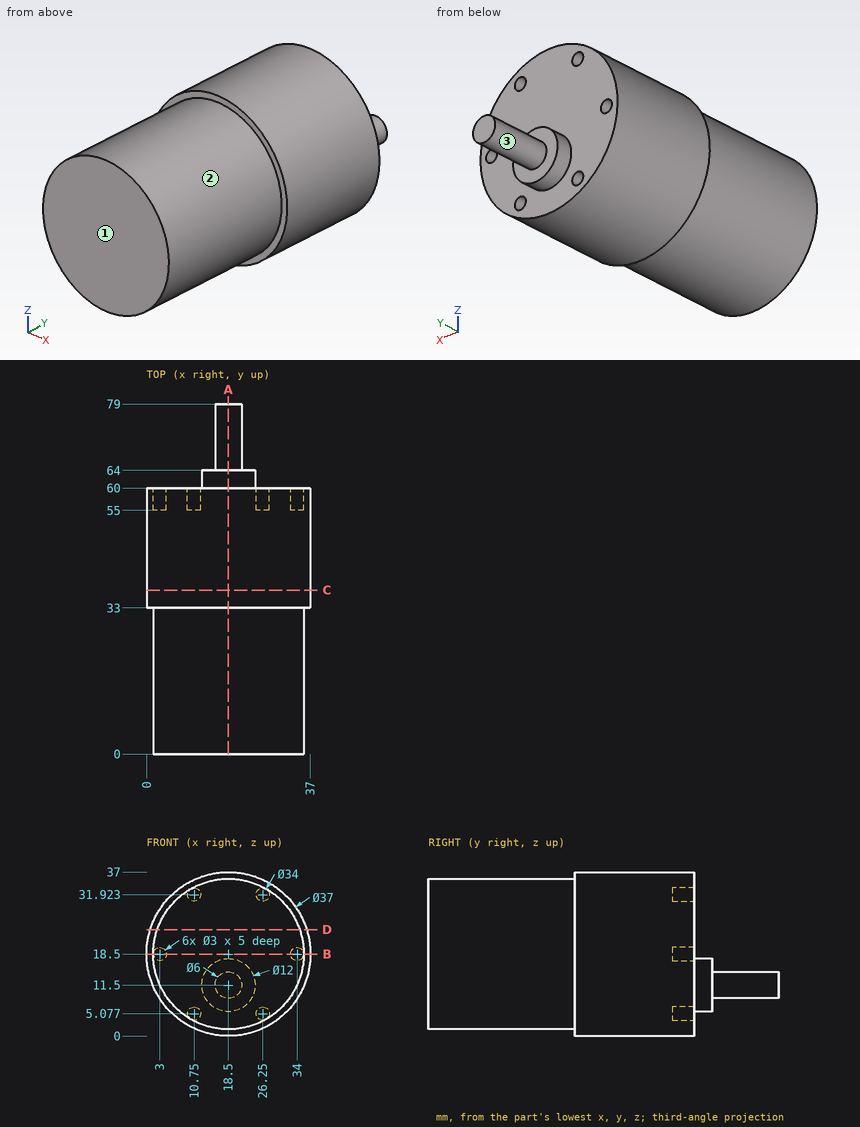
Could you check a few things on this drawing? It's one solid part, dimensions in mm from its lowest x, y, z. A direction names the side the tool comes from. Give positions to 0.01 mm unless a question says otherwise; leave off trailing zeros. Loops run counter-clockwise (first coordinate to the right, second up) from the corner with the lowest first, then second, coordinate; pieces in that order, holes last. Notation, with made-up numbers: M 21,-3.5 L 33,-3.5 A19 ccw 33,1.5 Z; hole C 75.5,49 d2. An arc over 180 degrees is marked long. One line per question, with ' | ' between items. Start each with the question number.
Q1. If we section it at A-A (x = 18.5): Please give me the cut outline in (y, z), plus the area to 3 significant figures.
Q2. If I drill on line 1 (X direction, y = 57.45, z = 18.5); line 2 (Z direction, x = 10, y = 57) (1 decimal); line 3 (Y direction, x = 9.5, z = 25), over which ranges is the centre line in solid material (lowest first)? Write a range as from..to.
Q3. If we section it at D-D (z = 24): Please give me the cut outline in (x, y) (1 decimal), plus the area to 3 significant figures.
Q4. If we section it at B-B (z = 18.5): Please give me the cut outline in (x, y).
Q5. For the marked faces 1, 2 and 3, which set-ups out of +Z, -Z, +X, -X, +Y, -Y let a thin tool reach every point of the face, with its end or its side?
Q6. For pin 1 Ø2.5 at (x, z) = (26, 32.5) entering from +Y; pin 2 Ø1.5 at (x, z) = (3, 19) entering from +Y; pin 3 Ø12 at (y, z) = (37.5, 8.5) entering from -X, each with a flat end and sliding along its axis, tell me the tip position at first contact or that it passes through.
Q7. If we section it at C-C (y = 37): Please give me the cut outline in (x, z), plus the area to 3 significant figures.
Computed:
1) outline: M 0,1.5 L 33,1.5 L 33,0 L 60,0 L 60,5.5 L 64,5.5 L 64,8.5 L 79,8.5 L 79,14.5 L 64,14.5 L 64,17.5 L 60,17.5 L 60,37 L 33,37 L 33,35.5 L 0,35.5 Z | area: 2,260 mm²
2) line 1: x = 0..1.5, 4.5..32.5, 35.5..37 | line 2: z = 2.1..3.8, 6.4..30.6, 33.2..34.9 | line 3: y = 0..60
3) outline: M 0.8,33 L 2.4,33 L 2.4,0 L 34.6,0 L 34.6,33 L 36.2,33 L 36.2,60 L 0.8,60 Z | area: 2,020 mm²
4) outline: M 0,33 L 1.5,33 L 1.5,0 L 35.5,0 L 35.5,33 L 37,33 L 37,60 L 35.5,60 L 35.5,55 L 32.5,55 L 32.5,60 L 4.5,60 L 4.5,55 L 1.5,55 L 1.5,60 L 0,60 Z
5) face 1: +Z, -Z, +X, -X, -Y | face 2: -Y | face 3: +Y
6) pin 1: stops at y = 60 | pin 2: stops at y = 55 | pin 3: stops at x = 0.44
7) outline: C 18.5,18.5 d37 | area: 1,080 mm²
